Source: CAD feature listing. Evaluate the final solid. Frame: model axes, mm. A direction names the side the tool comes from. Coordinates: 2 decimals unless noted, no trailing zeros. Loops run counter-clockwise (first coordinate to the right, second up) from the corner with the lowest first, then second, coordinate; pieces in that order, holes last.
from build123d import *

# Parameters (mm, degrees)
SKETCH1_R           = 5
SKETCH1_R_2         = 1.75
BOSS_EXTRUDE1_DEPTH = 4.5
BOSS_EXTRUDE2_START = -4.5
BOSS_EXTRUDE2_DEPTH = 4.5


with BuildPart() as part:
    # Sketch1 → Boss-Extrude1 (new body)
    # profile 1 of 3: a face of its own
    with BuildSketch(Plane.XY):
        with Locations((-11, 0)):
            Circle(SKETCH1_R)
        with Locations((-11, 0)):
            Circle(SKETCH1_R_2, mode=Mode.SUBTRACT)
    # profile 2 of 3: a face of its own
    with BuildSketch(Plane.XY):
        with BuildLine():
            ThreePointArc((-6, 0), (-7.464466094, -3.535533906), (-11, -5))
            Line((-11, -5), (11, -5))
            ThreePointArc((11, -5), (6, 0), (11, 5))
            Line((11, 5), (-11, 5))
            ThreePointArc((-11, 5), (-7.464466094, 3.535533906), (-6, 0))
        make_face()
    # profile 3 of 3: a face of its own
    with BuildSketch(Plane.XY):
        with Locations((11, 0)):
            Circle(SKETCH1_R)
        with Locations((11, 0)):
            Circle(SKETCH1_R_2, mode=Mode.SUBTRACT)
    extrude(amount=BOSS_EXTRUDE1_DEPTH)

    # Sketch2 → Boss-Extrude2 (add)
    with BuildSketch(Plane.XY.offset(4.5).offset(BOSS_EXTRUDE2_START)):
        with BuildLine():
            Line((49.180795902, 10.03), (46.363989199, 12.87))
            add(Edge.make_bspline(
                [(0, 5), (22.885517501, 10.707926651), (46.363989199, 12.87)],
                knots=[0, 0, 0, 1, 1, 1], degree=2))
            Line((0, 5), (11, 5))
            ThreePointArc((11, 5), (16, 0), (11, -5))
            Line((11, -5), (13.99, -5))
            Line((13.99, -5), (20.61, -1.48))
            add(Edge.make_bspline(
                [(42.27, 6), (30.146150748, 6.157348305), (20.61, -1.48)],
                knots=[0, 0, 0, 1, 1, 1], degree=2))
            Line((42.27, 6), (49.180795902, 10.03))
        make_face()
    extrude(amount=BOSS_EXTRUDE2_DEPTH)


solid = part.part
Q1. Line query: line 1 along Y through (x, z) = (-11, 2); line 2 along X through (y, z) = (-1.5, 2.15); line 3 along Y through (x, z) = (11, 2.6). Output: solid intervals per line, ascending.
Q2. Draft query along X for faces 3 (the flat face through (1, -5, 2)), 4 (the cylindrical face through (-9.331, 0.526, 2.218)), 5 (the flat face through (17.254, -3.265, 2.218)), 6 (the cylindrical face through (12.669, 0.526, 2.218)). Return one class per face: +X half, -X half, draft (parallel to the pull), parting line (faces both ways), or undercut.
Q3. Section B-B, the plane z = 2.1. Count the separate pieces of the cut face and the enclosed holes in it, plus the area to 3 significant figures.
Q4. Section A-A, the plane x = -6.5. Return the cut outline in (y, z).
Q5. Contact query for flat-ended pins moving along their axis: pin 1 Ø1.3 at (x, z) = (-7, 1.5) entering from +Y; pin 2 Ø2 at (y, z) = (2.5, 1.5) entering from -X. Output: stop coordinate, or through.
Q6. Access query for faces 1 (the flat face through (-5, 5, 2)), 2 (the flat face through (45.7, 8, 2.2)). Directions: +Z, -Z, +X, -X, +Y, -Y. A direction counts if a zero-diameter tool reaches every point of the face in a straight line with its end or side. Return the directions, or none.
Derived:
1. line 1: y = -5 to -1.75, 1.75 to 5
1. line 2: x = -15.77 to -11.9, -10.1 to 10.1, 11.9 to 20.57
1. line 3: y = -5 to -1.75, 1.75 to 7.53
2. face 3: draft
2. face 4: undercut
2. face 5: +X half
2. face 6: undercut
3. separate pieces: 1
3. enclosed holes: 2
3. area: 560 mm2
4. outline: (-5, 0) - (5, 0) - (5, 4.5) - (-5, 4.5) - close
5. pin 1: stops at y = 5
5. pin 2: stops at x = -15.77
6. face 1: +Z, -Z, -X, +Y
6. face 2: +Z, -Z, +X, -Y
